The model under review builds one solid part; all positions refer to its coordinate system, in mm. A direction names the side the tool comes from. Give positions to 0.01 mm unless a question says otherwise; leave off trailing zeros. Loops run counter-clockwise (first coordinate to the right, second up) from the corner with the lowest first, then second, coordinate; pieces in that order, holes last. Notation, with made-up numbers: M 72,83.5 L 86,83.5 A22 ccw 86,121.5 Z; hole C 41.5,-34 d9. An arc over 180 degrees is marked long. Write item = value, one per line. Start each with the question number.
1. We need section B-B on z = 6. Give the boundary of the cut face in (x, y).
2. Wall thickness on line 1 along X through (y, z) = (-14, 4); line 2 along Z through (x, y) = (-15, 42); line 3 along X through (y, z) = (36, 15): over which ranges is each line inside the solid? List them lowest first. Write a range as from..to.
3. For faces 5 (the face through (0, 32.1, 21)), 6 (the face through (18, 0, 11)), 7 (the face through (0, 20.1, 27)), list the 3-axis set-ups (+Z, -Z, +X, -X, +Y, -Y) from which the entire face can be reached by the end or side of a thin tool; tool diameter is ignored.
4. For pin 1 (4 mm diameter, centred on x = 6.5, y = 42, fed in from -Z); pin 2 (6.5 mm diameter, centred on x = -7.5, y = 3.5, fed in from +Z); pin 3 (14.5 mm diameter, centred on x = -9.5, z = 26.5, fed in from -Y), all flat-tipped, find the tip position at first contact; note any pin that passes through.
5. We need section C-C on y = 37. Give the boundary of the cut face in (x, z), then the cut area to 3 significant figures.
6. Draft analysis for pull direction Z (two halves, no side actions). For faces 1 (the face through (18, 50.1, 21)), 2 (the face through (0, -17, 12)), 3 (the face through (18, 40, 6)), 4 (the face through (-18, 40, 6)), state which applies: pulls with the +Z half, pulls with the -Z half, needs draft (parallel to the pull), parting line crosses it, or undercut.
7. We need section A-A on x = 20. Give the boundary of the cut face in (y, z).
8. We need section D-D on z = 20. Give the boundary of the cut face in (x, y).
from build123d import *

# Parameters (mm, degrees)
SZKIC1_W                    = 52
SZKIC1_H                    = 38
SZKIC1_R                    = 2.1
DODANIE_WYCI_GNI_CIE1_DEPTH = 12
SZKIC2_W                    = 32
SZKIC2_H                    = 22
WYTNIJ_WYCI_GNI_CIE1_DEPTH  = 3
SFAZOWANIE1_SIZE            = 3
DODANIE_WYCI_GNI_CIE2_DEPTH = 12
DODANIE_WYCI_GNI_CIE3_DEPTH = 30
SFAZOWANIE2_SIZE            = 1
SZKIC6_R                    = 2.1
WYTNIJ_WYCI_GNI_CIE2_DEPTH  = 84.534483897


with BuildPart() as part:
    # Szkic1 → Dodanie-wyciągnięcie1 (new body)
    with BuildSketch(Plane.XY):
        Rectangle(SZKIC1_W, SZKIC1_H)
        with Locations((20, 14.1)):
            Circle(SZKIC1_R, mode=Mode.SUBTRACT)
        with Locations(Location((20, -14.1, 0), (0, 0, 180))):
            Circle(SZKIC1_R, mode=Mode.SUBTRACT)
        with Locations((-20, -14.1)):
            Circle(SZKIC1_R, mode=Mode.SUBTRACT)
        with Locations(Location((-20, 14.1, 0), (0, 0, 180))):
            Circle(SZKIC1_R, mode=Mode.SUBTRACT)
    extrude(amount=DODANIE_WYCI_GNI_CIE1_DEPTH)

    # Szkic2 → Wytnij-wyciągnięcie1 (cut)
    with BuildSketch(Plane.XY.offset(12)):
        Rectangle(SZKIC2_W, SZKIC2_H)
    extrude(amount=-WYTNIJ_WYCI_GNI_CIE1_DEPTH, mode=Mode.SUBTRACT)

    # Sfazowanie1
    # the kernel refuses this chamfer: 3 mm, written as the material it takes off along each edge
    with BuildSketch(Plane(origin=(16, -11, 12), x_dir=(0, -0.9996219169112969, 0.02749587661058621), z_dir=(-1, 0, 0))) as sfazowanie1_piece_1_section:
        Polygon((SFAZOWANIE1_SIZE * 0.999621916911, -SFAZOWANIE1_SIZE * 0.0274958766106), (-SFAZOWANIE1_SIZE * 0.0274958766106, -SFAZOWANIE1_SIZE * 0.999621916911), (0, 0), align=None)
    sfazowanie1_piece_1 = extrude(amount=32, mode=Mode.PRIVATE)
    sfazowanie1_piece_1 = split(sfazowanie1_piece_1, bisect_by=Plane(origin=(0, -11.991212463, 9), z_dir=(0, 0, 1)), keep=Keep.TOP, mode=Mode.PRIVATE)
    add(sfazowanie1_piece_1, mode=Mode.SUBTRACT)
    with BuildSketch(Plane(origin=(16, 11, 12), x_dir=(0.9996219169112968, 0, 0.02749587661058619), z_dir=(0, -1, 0))) as sfazowanie1_piece_2_section:
        Polygon((SFAZOWANIE1_SIZE * 0.999621916911, -SFAZOWANIE1_SIZE * 0.0274958766106), (-SFAZOWANIE1_SIZE * 0.0274958766106, -SFAZOWANIE1_SIZE * 0.999621916911), (0, 0), align=None)
    sfazowanie1_piece_2 = extrude(amount=22, mode=Mode.PRIVATE)
    sfazowanie1_piece_2 = split(sfazowanie1_piece_2, bisect_by=Plane(origin=(16.991212463, 0, 9), z_dir=(0, 0, 1)), keep=Keep.TOP, mode=Mode.PRIVATE)
    add(sfazowanie1_piece_2, mode=Mode.SUBTRACT)
    with BuildSketch(Plane(origin=(-16, -11, 12), x_dir=(-0.9996219169112968, 0, 0.02749587661058619), z_dir=(0, 1, 0))) as sfazowanie1_piece_3_section:
        Polygon((SFAZOWANIE1_SIZE * 0.999621916911, -SFAZOWANIE1_SIZE * 0.0274958766106), (-SFAZOWANIE1_SIZE * 0.0274958766106, -SFAZOWANIE1_SIZE * 0.999621916911), (0, 0), align=None)
    sfazowanie1_piece_3 = extrude(amount=22, mode=Mode.PRIVATE)
    sfazowanie1_piece_3 = split(sfazowanie1_piece_3, bisect_by=Plane(origin=(-16.991212463, 0, 9), z_dir=(0, 0, 1)), keep=Keep.TOP, mode=Mode.PRIVATE)
    add(sfazowanie1_piece_3, mode=Mode.SUBTRACT)
    with BuildSketch(Plane(origin=(-16, 11, 12), x_dir=(0, 0.9996219169112969, 0.02749587661058621), z_dir=(1, 0, 0))) as sfazowanie1_piece_4_section:
        Polygon((SFAZOWANIE1_SIZE * 0.999621916911, -SFAZOWANIE1_SIZE * 0.0274958766106), (-SFAZOWANIE1_SIZE * 0.0274958766106, -SFAZOWANIE1_SIZE * 0.999621916911), (0, 0), align=None)
    sfazowanie1_piece_4 = extrude(amount=32, mode=Mode.PRIVATE)
    sfazowanie1_piece_4 = split(sfazowanie1_piece_4, bisect_by=Plane(origin=(0, 11.991212463, 9), z_dir=(0, 0, 1)), keep=Keep.TOP, mode=Mode.PRIVATE)
    add(sfazowanie1_piece_4, mode=Mode.SUBTRACT)
    with BuildSketch(Plane(origin=(16, 11, 12), x_dir=(0.9996219169112968, 0, 0.02749587661058619), z_dir=(0, -1, 0))) as sfazowanie1_piece_5a_section:
        Polygon((SFAZOWANIE1_SIZE * 0.999621916911, -SFAZOWANIE1_SIZE * 0.0274958766106), (-SFAZOWANIE1_SIZE * 0.0274958766106, -SFAZOWANIE1_SIZE * 0.999621916911), (0, 0), align=None)
    sfazowanie1_piece_5a = extrude(amount=29.715048964, mode=Mode.PRIVATE)
    sfazowanie1_piece_5a = split(sfazowanie1_piece_5a, bisect_by=Plane(origin=(16.991212463, -11, 11.014096999), z_dir=(0, -1, 0)), keep=Keep.TOP, mode=Mode.PRIVATE)
    sfazowanie1_piece_5a = split(sfazowanie1_piece_5a, bisect_by=Plane(origin=(16.991212463, -14.857524482, 9), z_dir=(0, 0, 1)), keep=Keep.TOP, mode=Mode.PRIVATE)
    with BuildSketch(Plane(origin=(23.715048964, -11, 12), x_dir=(0, -0.9996219169112969, 0.02749587661058621), z_dir=(-1, 0, 0))) as sfazowanie1_piece_5b_section:
        Polygon((SFAZOWANIE1_SIZE * 0.999621916911, -SFAZOWANIE1_SIZE * 0.0274958766106), (-SFAZOWANIE1_SIZE * 0.0274958766106, -SFAZOWANIE1_SIZE * 0.999621916911), (0, 0), align=None)
    sfazowanie1_piece_5b = extrude(amount=39.715048964, mode=Mode.PRIVATE)
    sfazowanie1_piece_5b = split(sfazowanie1_piece_5b, bisect_by=Plane(origin=(16, -11.991212463, 11.014096999), z_dir=(1, 0, 0)), keep=Keep.TOP, mode=Mode.PRIVATE)
    sfazowanie1_piece_5b = split(sfazowanie1_piece_5b, bisect_by=Plane(origin=(19.857524482, -11.991212463, 9), z_dir=(0, 0, 1)), keep=Keep.TOP, mode=Mode.PRIVATE)
    sfazowanie1_piece_5 = sfazowanie1_piece_5a & sfazowanie1_piece_5b
    add(sfazowanie1_piece_5, mode=Mode.SUBTRACT)
    with BuildSketch(Plane(origin=(-16, -18.715048964, 12), x_dir=(-0.9996219169112968, 0, 0.02749587661058619), z_dir=(0, 1, 0))) as sfazowanie1_piece_6a_section:
        Polygon((SFAZOWANIE1_SIZE * 0.999621916911, -SFAZOWANIE1_SIZE * 0.0274958766106), (-SFAZOWANIE1_SIZE * 0.0274958766106, -SFAZOWANIE1_SIZE * 0.999621916911), (0, 0), align=None)
    sfazowanie1_piece_6a = extrude(amount=29.715048964, mode=Mode.PRIVATE)
    sfazowanie1_piece_6a = split(sfazowanie1_piece_6a, bisect_by=Plane(origin=(-16.991212463, -11, 11.014096999), z_dir=(0, -1, 0)), keep=Keep.TOP, mode=Mode.PRIVATE)
    sfazowanie1_piece_6a = split(sfazowanie1_piece_6a, bisect_by=Plane(origin=(-16.991212463, -14.857524482, 9), z_dir=(0, 0, 1)), keep=Keep.TOP, mode=Mode.PRIVATE)
    with BuildSketch(Plane(origin=(16, -11, 12), x_dir=(0, -0.9996219169112969, 0.02749587661058621), z_dir=(-1, 0, 0))) as sfazowanie1_piece_6b_section:
        Polygon((SFAZOWANIE1_SIZE * 0.999621916911, -SFAZOWANIE1_SIZE * 0.0274958766106), (-SFAZOWANIE1_SIZE * 0.0274958766106, -SFAZOWANIE1_SIZE * 0.999621916911), (0, 0), align=None)
    sfazowanie1_piece_6b = extrude(amount=39.715048964, mode=Mode.PRIVATE)
    sfazowanie1_piece_6b = split(sfazowanie1_piece_6b, bisect_by=Plane(origin=(-16, -11.991212463, 11.014096999), z_dir=(-1, 0, 0)), keep=Keep.TOP, mode=Mode.PRIVATE)
    sfazowanie1_piece_6b = split(sfazowanie1_piece_6b, bisect_by=Plane(origin=(-19.857524482, -11.991212463, 9), z_dir=(0, 0, 1)), keep=Keep.TOP, mode=Mode.PRIVATE)
    sfazowanie1_piece_6 = sfazowanie1_piece_6a & sfazowanie1_piece_6b
    add(sfazowanie1_piece_6, mode=Mode.SUBTRACT)
    with BuildSketch(Plane(origin=(16, 18.715048964, 12), x_dir=(0.9996219169112968, 0, 0.02749587661058619), z_dir=(0, -1, 0))) as sfazowanie1_piece_7a_section:
        Polygon((SFAZOWANIE1_SIZE * 0.999621916911, -SFAZOWANIE1_SIZE * 0.0274958766106), (-SFAZOWANIE1_SIZE * 0.0274958766106, -SFAZOWANIE1_SIZE * 0.999621916911), (0, 0), align=None)
    sfazowanie1_piece_7a = extrude(amount=29.715048964, mode=Mode.PRIVATE)
    sfazowanie1_piece_7a = split(sfazowanie1_piece_7a, bisect_by=Plane(origin=(16.991212463, 11, 11.014096999), z_dir=(0, 1, 0)), keep=Keep.TOP, mode=Mode.PRIVATE)
    sfazowanie1_piece_7a = split(sfazowanie1_piece_7a, bisect_by=Plane(origin=(16.991212463, 14.857524482, 9), z_dir=(0, 0, 1)), keep=Keep.TOP, mode=Mode.PRIVATE)
    with BuildSketch(Plane(origin=(-16, 11, 12), x_dir=(0, 0.9996219169112969, 0.02749587661058621), z_dir=(1, 0, 0))) as sfazowanie1_piece_7b_section:
        Polygon((SFAZOWANIE1_SIZE * 0.999621916911, -SFAZOWANIE1_SIZE * 0.0274958766106), (-SFAZOWANIE1_SIZE * 0.0274958766106, -SFAZOWANIE1_SIZE * 0.999621916911), (0, 0), align=None)
    sfazowanie1_piece_7b = extrude(amount=39.715048964, mode=Mode.PRIVATE)
    sfazowanie1_piece_7b = split(sfazowanie1_piece_7b, bisect_by=Plane(origin=(16, 11.991212463, 11.014096999), z_dir=(1, 0, 0)), keep=Keep.TOP, mode=Mode.PRIVATE)
    sfazowanie1_piece_7b = split(sfazowanie1_piece_7b, bisect_by=Plane(origin=(19.857524482, 11.991212463, 9), z_dir=(0, 0, 1)), keep=Keep.TOP, mode=Mode.PRIVATE)
    sfazowanie1_piece_7 = sfazowanie1_piece_7a & sfazowanie1_piece_7b
    add(sfazowanie1_piece_7, mode=Mode.SUBTRACT)
    with BuildSketch(Plane(origin=(-23.715048964, 11, 12), x_dir=(0, 0.9996219169112969, 0.02749587661058621), z_dir=(1, 0, 0))) as sfazowanie1_piece_8a_section:
        Polygon((SFAZOWANIE1_SIZE * 0.999621916911, -SFAZOWANIE1_SIZE * 0.0274958766106), (-SFAZOWANIE1_SIZE * 0.0274958766106, -SFAZOWANIE1_SIZE * 0.999621916911), (0, 0), align=None)
    sfazowanie1_piece_8a = extrude(amount=39.715048964, mode=Mode.PRIVATE)
    sfazowanie1_piece_8a = split(sfazowanie1_piece_8a, bisect_by=Plane(origin=(-16, 11.991212463, 11.014096999), z_dir=(-1, 0, 0)), keep=Keep.TOP, mode=Mode.PRIVATE)
    sfazowanie1_piece_8a = split(sfazowanie1_piece_8a, bisect_by=Plane(origin=(-19.857524482, 11.991212463, 9), z_dir=(0, 0, 1)), keep=Keep.TOP, mode=Mode.PRIVATE)
    with BuildSketch(Plane(origin=(-16, -11, 12), x_dir=(-0.9996219169112968, 0, 0.02749587661058619), z_dir=(0, 1, 0))) as sfazowanie1_piece_8b_section:
        Polygon((SFAZOWANIE1_SIZE * 0.999621916911, -SFAZOWANIE1_SIZE * 0.0274958766106), (-SFAZOWANIE1_SIZE * 0.0274958766106, -SFAZOWANIE1_SIZE * 0.999621916911), (0, 0), align=None)
    sfazowanie1_piece_8b = extrude(amount=29.715048964, mode=Mode.PRIVATE)
    sfazowanie1_piece_8b = split(sfazowanie1_piece_8b, bisect_by=Plane(origin=(-16.991212463, 11, 11.014096999), z_dir=(0, 1, 0)), keep=Keep.TOP, mode=Mode.PRIVATE)
    sfazowanie1_piece_8b = split(sfazowanie1_piece_8b, bisect_by=Plane(origin=(-16.991212463, 14.857524482, 9), z_dir=(0, 0, 1)), keep=Keep.TOP, mode=Mode.PRIVATE)
    sfazowanie1_piece_8 = sfazowanie1_piece_8a & sfazowanie1_piece_8b
    add(sfazowanie1_piece_8, mode=Mode.SUBTRACT)

    # Szkic3 → Dodanie-wyciągnięcie2 (add)
    with BuildSketch(Plane.XY.offset(12)):
        Polygon((-10.2, 32.1), (10.2, 32.1), (10.2, 50.1), (26, 50.1), (26, 19), (-26, 19), (-26, 50.1), (-10.2, 50.1), align=None)
    extrude(amount=-DODANIE_WYCI_GNI_CIE2_DEPTH)

    # Szkic4 → Dodanie-wyciągnięcie3 (add)
    with BuildSketch(Plane.XY.offset(12)):
        Polygon((-26, 20.1), (26, 20.1), (26, 50.1), (10.2, 50.1), (10.2, 32.1), (-10.2, 32.1), (-10.2, 50.1), (-26, 50.1), align=None)
    extrude(amount=DODANIE_WYCI_GNI_CIE3_DEPTH)

    # Sfazowanie2
    sfazowanie2_edges = [part.edges().sort_by_distance(p)[0] for p in [
        (0, 20.1, 12),
    ]]
    chamfer(sfazowanie2_edges, length=SFAZOWANIE2_SIZE)

    # Szkic6 → Wytnij-wyciągnięcie2 (cut, through all)
    with BuildSketch(Plane(origin=(26, 0, 0), x_dir=(0, 0, -1), z_dir=(1, 0, 0))):
        with Locations((-36, 42.1)):
            Circle(SZKIC6_R)
        with Locations((-6, 42.1)):
            Circle(SZKIC6_R)
    extrude(amount=-WYTNIJ_WYCI_GNI_CIE2_DEPTH, mode=Mode.SUBTRACT)


solid = part.part
Final values:
q1.outline = M -26,-19 L 26,-19 L 26,40 L 10.2,40 L 10.2,32.1 L -10.2,32.1 L -10.2,40 L -26,40 Z; M -26,44.2 L -10.2,44.2 L -10.2,50.1 L -26,50.1 Z; M 10.2,44.2 L 26,44.2 L 26,50.1 L 10.2,50.1 Z; hole C -20,-14.1 d4.2; hole C -20,14.1 d4.2; hole C 20,-14.1 d4.2; hole C 20,14.1 d4.2
q2.line_1 = -26..-22.1, -17.9..17.9, 22.1..26
q2.line_2 = 0..3.9, 8.1..33.9, 38.1..42
q2.line_3 = -26..-10.2, 10.2..26
q3.face_5 = +Z, -Z, +Y
q3.face_6 = +Z
q3.face_7 = +Z, +X, -X, -Y
q4.pin_1 = through
q4.pin_2 = 9
q4.pin_3 = 20.1
q5.outline = M -26,0 L -10.2,0 L -10.2,42 L -26,42 Z; M 10.2,0 L 26,0 L 26,42 L 10.2,42 Z
q5.area = 1,330 mm²
q6.face_1 = needs draft
q6.face_2 = pulls with the +Z half
q6.face_3 = undercut
q6.face_4 = undercut
q7.outline = M -19,0 L -16.2,0 L -16.2,12 L -19,12 Z; M -12,0 L 12,0 L 12,12 L -12,12 Z; M 16.2,0 L 50.1,0 L 50.1,42 L 20.1,42 L 20.1,13 L 19.1,12 L 16.2,12 Z; hole C 42.1,6 d4.2; hole C 42.1,36 d4.2
q8.outline = M -26,20.1 L 26,20.1 L 26,50.1 L 10.2,50.1 L 10.2,32.1 L -10.2,32.1 L -10.2,50.1 L -26,50.1 Z
